```python
from build123d import *

# Parameters (mm, degrees)
SKETCH1_R           = 2
BOSS_EXTRUDE1_DEPTH = 1
BOSS_EXTRUDE2_DEPTH = 70
CUT_EXTRUDE1_DEPTH  = 70
FILLET1_R           = 6
FILLET2_R           = 6


with BuildPart() as part:
    # Sketch1 → Boss-Extrude1 (new body)
    with BuildSketch(Plane(origin=(0, 0, 0), x_dir=(1, 0, 0), z_dir=(0, 1, 0))):
        with BuildLine():
            Line((-12.999999999999979, -60.5), (12.99999999999998, -60.5))
            ThreePointArc((12.99999999999998, -60.5), (15.121320343559649, -59.62132034355964), (16, -57.49999999999997))
            Line((16, -57.49999999999997), (16, 57.49999999999997))
            ThreePointArc((16, 57.49999999999997), (15.121320343559649, 59.62132034355964), (12.99999999999998, 60.5))
            Line((12.99999999999998, 60.5), (-12.999999999999979, 60.5))
            ThreePointArc((-12.999999999999979, 60.5), (-15.121320343559644, 59.62132034355963), (-16, 57.49999999999997))
            Line((-16, 57.49999999999997), (-16, -57.49999999999997))
            ThreePointArc((-16, -57.49999999999997), (-15.121320343559649, -59.62132034355964), (-12.999999999999979, -60.5))
        make_face()
        with Locations(Location((-12, 56, 0), (0, 0, 270))):
            Circle(SKETCH1_R, mode=Mode.SUBTRACT)
        with Locations(Location((12, 56, 0), (0, 0, 90))):
            Circle(SKETCH1_R, mode=Mode.SUBTRACT)
        with Locations(Location((12, -56, 0), (0, 0, 270))):
            Circle(SKETCH1_R, mode=Mode.SUBTRACT)
        with Locations(Location((-12, -56, 0), (0, 0, 90))):
            Circle(SKETCH1_R, mode=Mode.SUBTRACT)
    extrude(amount=BOSS_EXTRUDE1_DEPTH)

    # Sketch2 → Boss-Extrude2 (add)
    with BuildSketch(Plane.XY.offset(20.499999999999996)):
        Polygon((-23.633274615316285, 1), (20.533692341844997, 1), (40.67208349009961, 25.000000000000004), (41.43812793321859, 24.357212390313464), (20.999999999999996, 0), (-24, -9.1e-16), (-28.999999999999993, 4.237089446732834), (-28.353495949190116, 4.9999999999999964), align=None)
    extrude(amount=-BOSS_EXTRUDE2_DEPTH)

    # Sketch3 → Cut-Extrude1 (cut)
    with BuildSketch(Plane.XZ):
        Polygon((20.999999999999996, 20.499999999999996), (20.999999999999996, 20.109633851053125), (40.672083490099595, 3.6412886727309868), (40.67208349009961, 20.499999999999993), align=None)
        Polygon((20.999999999999996, 20.499999999999996), (20.533692341844997, 20.499999999999996), (20.999999999999993, 20.109633851053125), align=None)
        Polygon((40.67208349009961, 20.499999999999993), (40.67208349009961, 3.6412886727309868), (41.43812793321859, 2.9999999999999964), (41.43812793321859, 20.499999999999993), align=None)
        Polygon((41.43812793321859, -32.00000000000001), (40.67208349009961, -32.64128867273098), (40.67208349009961, -49.50000000000001), (41.43812793321859, -49.50000000000001), align=None)
        Polygon((40.67208349009961, -32.64128867273098), (20.999999999999996, -49.10963385105313), (20.999999999999996, -49.5), (40.67208349009961, -49.50000000000001), align=None)
        Polygon((-24, -49.50000000000001), (-23.633274615316285, -49.50000000000001), (-24.00000000000002, -48.30416943816782), align=None)
        Polygon((-24, -49.50000000000001), (-24, -48.30416943816781), (-28.353495949190155, -34.108142317373115), (-28.353495949190116, -49.5), align=None)
        Polygon((-28.353495949190116, -49.5), (-28.353495949190116, -34.10814231737311), (-28.999999999999993, -32.00000000000001), (-28.999999999999993, -49.5), align=None)
        Polygon((-24.00000000000002, 19.304169438167804), (-23.633274615316285, 20.499999999999996), (-24, 20.499999999999996), align=None)
        Polygon((-28.353495949190116, 5.108142317373225), (-24.00000000000002, 19.304169438167804), (-24, 20.499999999999993), (-28.353495949190116, 20.499999999999996), align=None)
        Polygon((-28.999999999999993, 2.9999999999999964), (-28.353495949190116, 5.108142317373225), (-28.353495949190116, 20.499999999999996), (-28.999999999999993, 20.499999999999996), align=None)
        Polygon((20.999999999999996, -49.10963385105313), (20.533692341844997, -49.50000000000001), (20.999999999999996, -49.50000000000001), align=None)
    extrude(amount=-CUT_EXTRUDE1_DEPTH, mode=Mode.SUBTRACT)

    # Fillet1
    fillet1_edges = [part.edges().sort_by_distance(p)[0] for p in [
        (-23.633274615316285, 1, -14.500000000000004),
        (20.533692341844997, 1, -14.500000000000004),
    ]]
    fillet(fillet1_edges, radius=FILLET1_R)

    # Fillet2
    fillet2_edges = [part.edges().sort_by_distance(p)[0] for p in [
        (-24, -9.1e-16, -14.50000000000001),
        (20.999999999999996, 0, -14.500000000000004),
    ]]
    fillet(fillet2_edges, radius=FILLET2_R)


solid = part.part
```
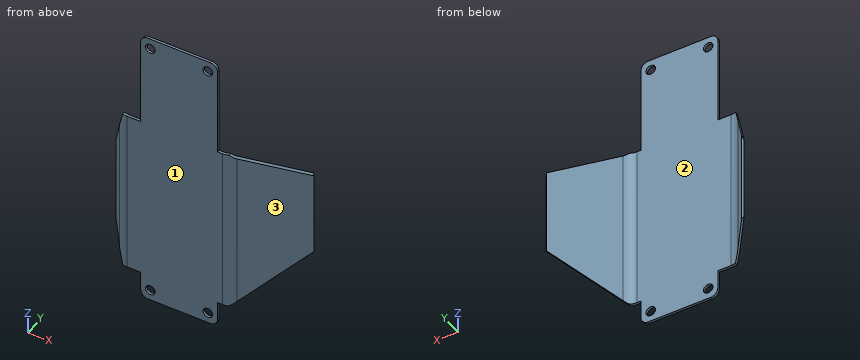
Part model, mm, in its own coordinate system. Face numbers are marked on the shaded views. Coordinates: 2 decimals unless noted, no trailing zeros. Order: outer loops, then holes, each group sorted by start corner. A loop starts at its lowest first (then second) coordinate and runs counter-clockwise, first axis right, second up. Notation, with made-up numbers: (6, -31.75) - (15, -31.75) arc R14 cw to (15, -8.75) - close; hole circle Ø3 at (86.5, 38.25). An arc over 180 degrees is marked (long way). Return JSON: item names as keys, results as strings. Group by question number.
Item 1: Pull direction X, two halves, no side cores. Call the marked faces 1, 2 and 3: pulls with the +X half, pulls with the -X half, needs draft (parallel to the pull), parting line crosses it, or undercut.
Item 2: Cut at A-A (z = -56). List the corners of the cut face in (x, y), plus the area to 3 significant figures.
Item 3: Cut at C-C (x = 1). List the corners of the cut face in (y, z), plus the area to 3 significant figures.
Item 4: Cut at D-D (y = 9.5). List the corners of the cut face in (x, z), plus the area to 3 significant figures.
Item 5: Drill centre lines: probe 1 along X at (y, z) = (0.5, -56); probe 2 along Y at (x, z) = (-14, -44.5); probe 3 along X at (y, z) = (3.5, -3). Where is each one in solid material? Low to high. Write a range as from..to.
Item 6: Cut at B-B (z = -19.5). List the corners of the cut face in (x, y).
Item 7: Pin check, flat tips, straight feed: pin 1 (6 mm diameter, centred on x = 11, z = -2, fed in from +Y); pin 2 (1.9 mm diameter, centred on x = 19, y = 1, fed in from +Z); pin 3 (2 mm diameter, centred on y = 9.5, z = -4.5, fed in from -X); pin 4 (4 mm diameter, centred on x = -13.5, y = 3.5, fed in from -Z). Stop position of each tip, or through.
Check values:
{
 "1": {"face 1": "needs draft", "face 2": "undercut", "face 3": "pulls with the +X half"},
 "2": {"outline": "(-16, 0) - (-14, 0) - (-14, 1) - (-16, 1) - close; (-10, 0) - (10, 0) - (10, 1) - (-10, 1) - close; (14, 0) - (16, 0) - (16, 1) - (14, 1) - close", "area": "24.0 mm2"},
 "3": {"outline": "(0, -60.5) - (1, -60.5) - (1, 60.5) - (0, 60.5) - close", "area": "121 mm2"},
 "4": {"outline": "(27.67, -43.53) - (28.97, -42.44) - (28.97, 13.44) - (27.67, 14.53) - close", "area": "74.4 mm2"},
 "5": {"probe 1": "x = -16..-14, -10..10, 14..16", "probe 2": "y = 0..1", "probe 3": "x = -28.13..-26.58, 22.63..23.94"},
 "6": {"outline": "(-29, 4.24) - (-25.68, 1.42) arc R6 ccw to (-21.8, 0) - (18.2, 0) arc R6 ccw to (22.8, 2.14) - (41.44, 24.36) - (40.67, 25) - (22.33, 3.14) arc R6 cw to (17.74, 1) - (-21.43, 1) arc R6 cw to (-25.31, 2.42) - (-28.35, 5) - close"},
 "7": {"pin 1": "stops at y = 1", "pin 2": "stops at z = 20.5", "pin 3": "stops at x = 26.83", "pin 4": "passes through"}
}
